from build123d import *

# Parameters (mm, degrees)
MODEL_R             = 2.5
MODEL_R_2           = 2.6
MODEL_R_3           = 2.55
BOSS_EXTRUDE1_DEPTH = 6.35


with BuildPart() as part:
    # Model → Boss-Extrude1 (new body)
    with BuildSketch(Plane.XY):
        Polygon((691.840616937, 302.611489719), (368.840616937, 302.611489719), (368.840616937, 447.611489719), (345.840616937, 447.611489719), (345.840616937, 534.611489719), (368.840616937, 534.611489719), (368.840616937, 644.611489719), (691.840616937, 644.611489719), align=None)
        with Locations((355.840616937, 514.611489719)):
            Circle(MODEL_R, mode=Mode.SUBTRACT)
        with Locations((355.840616937, 492.611489719)):
            Circle(MODEL_R, mode=Mode.SUBTRACT)
        with Locations((355.840616937, 467.611489719)):
            Circle(MODEL_R, mode=Mode.SUBTRACT)
        with Locations((430, 570)):
            Circle(MODEL_R_2, mode=Mode.SUBTRACT)
        with Locations((494.9, 570)):
            Circle(MODEL_R_2, mode=Mode.SUBTRACT)
        with Locations((451.840616937, 483.611489719)):
            Circle(MODEL_R, mode=Mode.SUBTRACT)
        with Locations((521.840616937, 483.611489719)):
            Circle(MODEL_R, mode=Mode.SUBTRACT)
        with Locations((601.840616937, 483.611489719)):
            Circle(MODEL_R, mode=Mode.SUBTRACT)
        with Locations((585, 570)):
            Circle(MODEL_R_2, mode=Mode.SUBTRACT)
        with Locations((649.9, 570)):
            Circle(MODEL_R_2, mode=Mode.SUBTRACT)
        with Locations((430, 388.410571956)):
            Circle(MODEL_R_2, mode=Mode.SUBTRACT)
        with Locations((494.9, 388.410571956)):
            Circle(MODEL_R_2, mode=Mode.SUBTRACT)
        with Locations((585.843810025, 411.289923372)):
            Circle(MODEL_R_3, mode=Mode.SUBTRACT)
        with Locations((640.843810025, 411.289923372)):
            Circle(MODEL_R_3, mode=Mode.SUBTRACT)
        with Locations((585.843810025, 356.289923372)):
            Circle(MODEL_R_3, mode=Mode.SUBTRACT)
        with Locations((640.843810025, 356.289923372)):
            Circle(MODEL_R_3, mode=Mode.SUBTRACT)
    extrude(amount=-BOSS_EXTRUDE1_DEPTH)


solid = part.part
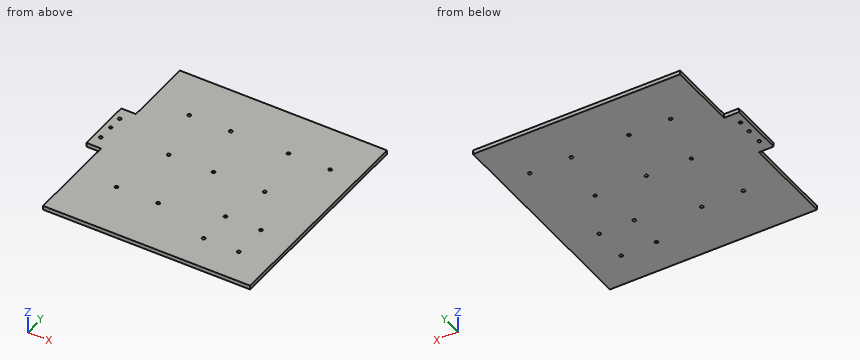
For this review, take the finished solid that the model builds, in its own axes (mm). Round coordinates to 2 decimals unless told otherwise and drop trailing zeros. Loops run counter-clockwise (first coordinate to the right, second up) from the corner with the lowest first, then second, coordinate; pieces in that order, holes last. Notation, with made-up numbers: (-19, 67) - (-10, 67) arc R36 ccw to (-10, 102) - close; hole circle Ø11 at (45.5, 70). An arc over 180 degrees is marked (long way). One line per question, with ' | ' between items.
Q1. For line 1 along X through (y, z) = (570, -4); line 2 along X through (y, z) = (409.5, -5.25); line 3 along Y through (x, z) = (494.9, -4.5), list the stretches that pass through material, from the lowest coordinate up. Write a range as [from, to].
Taken from the geometry:
line 1: x = [368.84, 427.4], [432.6, 492.3], [497.5, 582.4], [587.6, 647.3], [652.5, 691.84] | line 2: x = [368.84, 584.03], [587.66, 639.03], [642.66, 691.84] | line 3: y = [302.61, 385.81], [391.01, 567.4], [572.6, 644.61]
Q2. For pin 1 (4.5 mm diameter, centred on x = 430, y = 388.41, fed in from -Z); pin 2 (2 mm diameter, centred on x = 447, y = 507.5, fed in from +Z); pin 3 (1 mm diameter, centred on y = 429, z = -2.5, fed in from -X); pin 4 (3 mm diameter, centred on x = 357, z = -3.5, fed in from +Y), all flat-tipped, find the tip position at first contact; note any pin that passes through.
Taken from the geometry:
pin 1: passes through | pin 2: stops at z = 0 | pin 3: stops at x = 368.84 | pin 4: stops at y = 534.61
Q3. Take a section at A-A (z = -3.5). State how many separate pieces and enclosed holes the cut face has, and give its area (3 significant figures).
Taken from the geometry:
separate pieces: 1 | enclosed holes: 16 | area: 112,000 mm²
Q4. Take a section at B-B (y = 555.5). Give the boundary of the cut face in (x, z).
Taken from the geometry:
outline: (368.84, -6.35) - (691.84, -6.35) - (691.84, 0) - (368.84, 0) - close
